from build123d import *

# Parameters (mm, degrees)
BOSS_EXTRUDE1_DEPTH      = 2
BOSS_EXTRUDE1_DEPTH_BACK = 1


with BuildPart() as part:
    # Sketch1 → Boss-Extrude1 (new, two sides: drawn at the far end of the back side and taken through both)
    with BuildSketch(Plane.XY.offset(-BOSS_EXTRUDE1_DEPTH_BACK)):
        Polygon((98.82804668, 60.344291492), (98.82804668, 98.844291492), (60.32804668, 98.844291492), (60.32804668, 101.844291492), (40.32804668, 101.844291492), (40.32804668, 98.844291492), (1.82804668, 98.844291492), (1.82804668, 60.344291492), (-1.17195332, 60.344291492), (-1.17195332, 40.344291492), (1.82804668, 40.344291492), (1.82804668, 1.844291492), (40.32804668, 1.844291492), (40.32804668, -1.155708508), (60.32804668, -1.155708508), (60.32804668, 1.844291492), (98.82804668, 1.844291492), (98.82804668, 40.344291492), (101.82804668, 40.344291492), (101.82804668, 60.344291492), align=None)
    extrude(amount=BOSS_EXTRUDE1_DEPTH + BOSS_EXTRUDE1_DEPTH_BACK)


solid = part.part
Input: part model. Units: mm. Frame: model coordinates. A direction names the side the tool comes from. Coordinates: 2 decimals unless noted, no trailing zeros. Order: outer loops, then holes, each group sorted by start corner. A loop starts at its lowest first (then second) coordinate and runs counter-clockwise, first axis right, second up. Notation, with made-up numbers: M 42,-22 L 86,-22 A21 ccw 86,-15 Z; hole C 87.25,56.25 d5. An arc over 180 degrees is marked long. Write item = value, one per line. Start each with the question number.
(1) Section B-B on x = 6. Output: boundary loops of the cut face in (y, z).
(2) Line query: line 1 along Y through (x, z) = (88.5, 0.3); line 2 along X through (y, z) = (63.5, 1.8). Output: solid intervals per line, ascending. Write a range as [from, to].
(3) Section A-A on z = 1.5. Output: boundary loops of the cut face in (x, y), and give its area (3 significant figures).
(4) First-contact query: P1, Ø1.5, axis at y = 101, z = 1, coming from the -X side; P2, Ø1.5, axis at y = 14, z = 1, coming from the -X side; P3, Ø0.9, axis at y = 72, z = 0, coming from the +X side. Flat tips, straight axial feed; report the tip coordinate or a pass-through.
(5) Section C-C on y = 33. Output: boundary loops of the cut face in (x, z).
(6) Reachability of faces 1 (the flat face through (0, 40.344, 0)), 2 (the flat face through (98.828, 79, 0)), 3 (the flat face through (60.328, 0, 0)), 4 (the flat face through (40.328, 100, 0)) from +Z, -Z, +X, -X, +Y, -Y: full face, straight path, thin tool, end or side. Return the list, or none.
Result set:
q1.outline = M 1.84,-1 L 98.84,-1 L 98.84,2 L 1.84,2 Z
q2.line_1 = [1.84, 98.84]
q2.line_2 = [1.83, 98.83]
q3.outline = M -1.17,40.34 L 1.83,40.34 L 1.83,1.84 L 40.33,1.84 L 40.33,-1.16 L 60.33,-1.16 L 60.33,1.84 L 98.83,1.84 L 98.83,40.34 L 101.83,40.34 L 101.83,60.34 L 98.83,60.34 L 98.83,98.84 L 60.33,98.84 L 60.33,101.84 L 40.33,101.84 L 40.33,98.84 L 1.83,98.84 L 1.83,60.34 L -1.17,60.34 Z
q3.area = 9,650 mm²
q4.P1 = 40.33
q4.P2 = 1.83
q4.P3 = 98.83
q5.outline = M 1.83,-1 L 98.83,-1 L 98.83,2 L 1.83,2 Z
q6.face_1 = +Z, -Z, -X, -Y
q6.face_2 = +Z, -Z, +X, +Y
q6.face_3 = +Z, -Z, +X, -Y
q6.face_4 = +Z, -Z, -X, +Y
